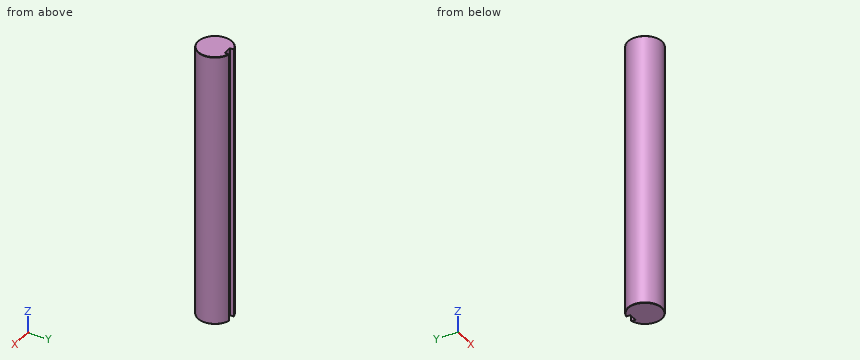
```python
from build123d import *

# Parameters (mm, degrees)
BOSS_EXTRUDE1_DEPTH      = 38.1
BOSS_EXTRUDE1_DEPTH_BACK = 38.1
CHAMFER1_SIZE            = 0.09525


with BuildPart() as part:
    # Sketch3 → Boss-Extrude1 (new body, two sides)
    with BuildSketch(Plane.XY) as boss_extrude1_sk:
        with BuildLine():
            Line((-1.1938, 3.416649849), (-1.1938, 4.610449849))
            ThreePointArc((-1.1938, 4.610449849), (0, -4.7625), (1.1938, 4.610449849))
            Line((1.1938, 4.610449849), (1.1938, 3.416649849))
            Line((1.1938, 3.416649849), (-1.1938, 3.416649849))
        make_face()
    extrude(amount=BOSS_EXTRUDE1_DEPTH)
    extrude(boss_extrude1_sk.sketch, amount=-BOSS_EXTRUDE1_DEPTH_BACK)

    # Chamfer1
    chamfer1_edges = [part.edges().sort_by_distance(p)[0] for p in [
        (0, -4.7625, -38.1),
        (0, -4.7625, 38.1),
    ]]
    chamfer(chamfer1_edges, length=CHAMFER1_SIZE)


solid = part.part
```
Input: part model. Units: mm. Frame: model coordinates. Coordinates: 2 decimals unless noted, no trailing zeros. Loops run counter-clockwise (first coordinate to the right, second up) from the corner with the lowest first, then second, coordinate; pieces in that order, holes last. Notation, with made-up numbers: (48, -29) - (91, -29) arc R21 cw to (91, -3) - close; hole circle Ø9 at (-17, 8.5). An arc over 180 degrees is marked (long way). Answer in a Markdown table with one row per item.
(1) Pin query (flat end, axial travel): P1, Ø1, axis at y = 3.5, z = 10, coming from the +X side; P2, Ø1.2, axis at x = 0.5, z = -8, coming from the +Y side; P3, Ø3, axis at y = 3, z = 8, coming from the -X side. Return the tip coordinate at first contact, or that it passes through.
Model answer:
| item | result |
|---|---|
| P1 | stops at x = 3.7 |
| P2 | stops at y = 3.42 |
| P3 | stops at x = -4.52 |
(2) Cut plane A-A on x = 0. Output: boundary loops of the cut face in (y, z), plus the area to 3 significant figures.
Model answer:
| item | result |
|---|---|
| outline | (-4.76, -38) - (-4.67, -38.1) - (3.42, -38.1) - (3.42, 38.1) - (-4.67, 38.1) - (-4.76, 38) - close |
| area | 623 mm² |
(3) Cut plane B-B on z = -32. Output: boundary loops of the cut face in (x, y) (1 decimal).
Model answer:
| item | result |
|---|---|
| outline | (-1.2, 3.4) - (-1.2, 4.6) arc R4.8 ccw (long way) to (1.2, 4.6) - (1.2, 3.4) - close |
(4) Material intervals for L1, parallel to Y at x = 1, z = 30.5; L2, parallel to X at y = -1, z = 16; L3, parallel to X at y = 0.25, z = -28.5, sorted ascending. Write a range as from..to.
Model answer:
| item | result |
|---|---|
| L1 | y = -4.66..3.42 |
| L2 | x = -4.66..4.66 |
| L3 | x = -4.76..4.76 |
